Could you check a few things on this drawing? It's one solid part, dimensions in mm from its lowest x, y, z. A direction names the side the tool comes from. Give positions to 0.01 mm unless a question says otherwise; leave off trailing zeros. Answer as CSV lines item,"result". Start each with the question number.
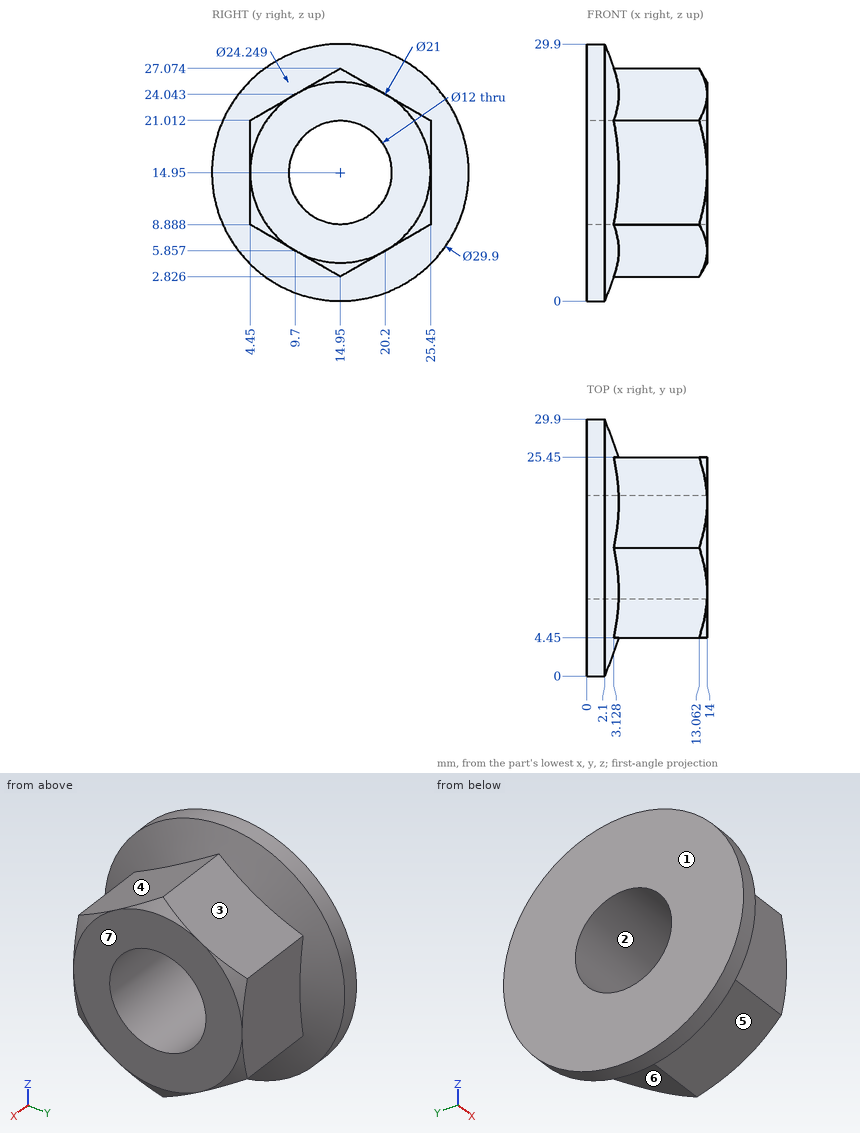
1) I'm going to push flat-ended pins straight in: P1, Ø3, axis at y = 3.5, z = 10, coming from the +X side (1 decimal); P2, Ø6, axis at x = 9, y = 5, coming from the -Z side; P3, Ø1.5, axis at x = 9.5, y = 16.5, coming from the +Z side. Where does each tip first touch, or does it pass through?
2) On a 3-axis mill with a long thin cutter (end or side, diameter ignored), from which of +Z, -Z, +X, -X, +Y, -Y can I reach the whole of each face in a straight line? I mean the marked faces 4, 5, 6 and 7. Say none if no direction works.
3) Thinking about a two-plate mould opening in Z: for the marked faces 1, 2 and 3, which applies, released by +Z, released by -Z, zero draft, split by the parting line, or undercut?
4) I need wall thicknesses on L1, parallel to Y at x = 8.75, z = 14.95; L2, parallel to Z at x = 9, y = 20.5 (1 decimal); L3, parallel to Y at x = 1.25, z = 1.75 (1 decimal). Which ranges of each line are inside material? Lowest first, please. Write a range as from..to.
Values found:
1,P1,"stops at x = 13.7"
1,P2,"stops at z = 6.84"
1,P3,"stops at z = 26.61"
2,face 4,"+Z, +X, -Y"
2,face 5,"-Z, +X, -Y"
2,face 6,"-Z, +X, +Y"
2,face 7,"+Z, -Z, +X, +Y, -Y"
3,face 1,"zero draft"
3,face 2,"undercut"
3,face 3,"released by +Z"
4,L1,"y = 4.45..8.95, 20.95..25.45"
4,L2,"z = 6..12.7, 17.2..23.9"
4,L3,"y = 7.9..22"
